Part model, mm, in its own coordinate system. Coordinates: 2 decimals unless noted, no trailing zeros. Loops run counter-clockwise (first coordinate to the right, second up) from the corner with the lowest first, then second, coordinate; pieces in that order, holes last. Notation, with made-up numbers: M 30,-21 L 68,-21 A15 ccw 68,-2 Z; hole C 66,86 d2. An arc over 180 degrees is marked long. Answer as a JSON object with one key per item and string values. Group by question number.
1. Saw through at A-A on y = 1.95. Write the cut outline in (x, z).
2. Drill centre lines: L1, parallel to Z at x = 0, y = 2.9; L2, parallel to X at y = 1.85, z = -137.5; L3, parallel to Z at x = -1.25, y = 1.75. Where is each one in solid material? Low to high.
3. Saw through at B-B on x = 0. Write the cut outline in (y, z).
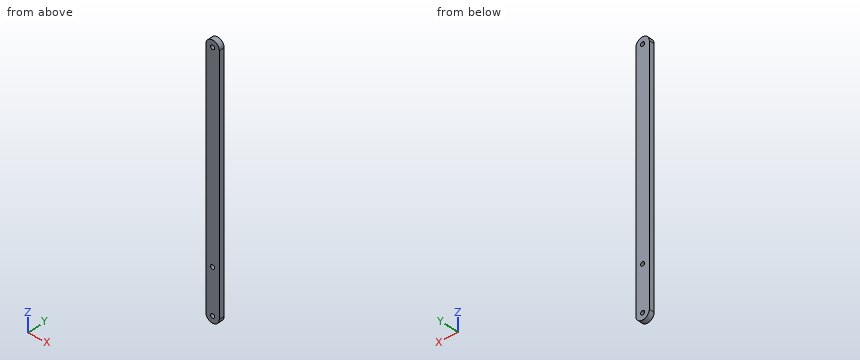
Autodesk Inventor part; units mm, degrees
ref_plane "YZ Plane" through (0, 0, 0) normal (1, 0, 0) x (0, 1, 0)
ref_plane "XZ Plane" through (0, 0, 0) normal (0, 1, 0) x (-1, 0, 0)
ref_plane "XY Plane" through (0, 0, 0) normal (0, 0, 1) x (1, 0, 0)
sketch "Szkic3" plane through (0, 0, 0) normal (0, 1, 0) x (-1, 0, 0)
  line L0 (0, -145) -> (0, -145)
  line L1 (7.5, -137.5) -> (7.5, 137.5)
  line L2 (0, 145) -> (0, 145)
  line L3 (-7.5, 137.5) -> (-7.5, -137.5)
  circle A0 centre (0, 137.5) radius 2.25
  circle A1 centre (0, -137.5) radius 2.25
  circle A2 centre (0, -87.5) radius 2.25
  arc A3 (7.5, 137.5) -> (0, 145) centre (0, 137.5) ccw
  arc A4 (0, 145) -> (-7.5, 137.5) centre (0, 137.5) ccw
  arc A5 (0, -145) -> (7.5, -137.5) centre (0, -137.5) ccw
  arc A6 (-7.5, -137.5) -> (0, -145) centre (0, -137.5) ccw
  point P0 (0, 0)
  point P1 (7.5, 145)
  point P2 (7.5, -145)
  point P3 (-7.5, 145)
  point P4 (0, 145)
  point P5 (7.1121, 137.5)
  point P6 (-7.1121, 137.5)
  point P7 (7.1121, -137.5)
  point P8 (0, -145)
  point P9 (-7.1121, -137.5)
  point P10 (0, 145)
  dimension "d11" = 15
  dimension "d12" = 290
  dimension "d13" = 4.5
  dimension "d14" = 4.5
  dimension "d15" = 4.5
  dimension "d16" = 7.5
  dimension "d17" = 7.5
extrude "Wyciągnięcie proste2" add sketch "Szkic3" along normal blind 6
properties part number "GraspArm"
Outcome:
{
 "1": {"outline": "M -7.5,-137.5 A7.5 ccw 7.5,-137.5 L 7.5,137.5 A7.5 ccw -7.5,137.5 Z; hole C 0,-137.5 d4.5; hole C 0,-87.5 d4.5; hole C 0,137.5 d4.5"},
 "2": {"L1": "z = -145 to -139.75, -135.25 to -89.75, -85.25 to 135.25, 139.75 to 145", "L2": "x = -7.5 to -2.25, 2.25 to 7.5", "L3": "z = -144.9 to -139.37, -135.63 to -89.37, -85.63 to 135.63, 139.37 to 144.9"},
 "3": {"outline": "M 0,-145 L 6,-145 L 6,-139.75 L 0,-139.75 Z; M 0,-135.25 L 6,-135.25 L 6,-89.75 L 0,-89.75 Z; M 0,-85.25 L 6,-85.25 L 6,135.25 L 0,135.25 Z; M 0,139.75 L 6,139.75 L 6,145 L 0,145 Z"}
}
